The model under review builds one solid part; all positions refer to its coordinate system, in mm. Round coordinates to 2 decimals unless told otherwise and drop trailing zeros. Order: outer loops, then holes, each group sorted by start corner. A loop starts at its lowest first (then second) coordinate and runs counter-clockwise, first axis right, second up. Notation, with made-up numbers: M 45.5,81 L 91.5,81 A23 cw 91.5,105 Z; hole C -33.5,-18.5 d4. An arc over 180 degrees is marked long. Answer as a JSON object with one key per item and string values. Group by question number.
1. Add section A-A on x = 0. State the section outline as (y, z) points.
2. Add section D-D on z = 11.5. State the section outline as (x, y) points, and give its area (3 significant figures).
3. Add section B-B on y = 7. State the section outline as (x, z) points.
4. Clearance check with a flat-ended pin moving along its axis: P1, Ø4, axis at x = 0, z = -20, coming from the +Y side. State where the tip first meets the part, or that it passes through.
5. To check wall thickness, follow probe 1 along Z at (x, y) = (0, 7.8); probe 2 along Z at (x, y) = (0, 3.3); probe 3 along Y at (x, z) = (-5.75, -29.5). State the ranges of each line that lie inside material, in increasing order. Write a range as [from, to].
Autodesk Inventor part; units mm, degrees
ref_plane "to_block_XY" through (0, 9.5, 0) normal (0, 0, 1) x (1, 0, 0)
ref_plane "to_block_YZ" through (0, 9.5, 0) normal (1, 0, 0) x (0, 1, 0)
ref_plane "to_block_ZX" through (0, 9.5, 0) normal (0, 1, 0) x (0, 0, 1)
sketch "Sketch_12" plane through (0, 0, 0) normal (0, 0, 1) x (1, 0, 0)
  line L0 (-7.5, 9.2) -> (-7.5, 8.7239)
  line L1 (-7.5, 8.7239) -> (-6.94, 8.4006)
  arc A0 (-6.2177, 7.6) -> (-6.94, 8.4006) centre (-7.815, 6.885) ccw
  line L2 (-6.2177, 7.6) -> (-5, 7.6)
  line L3 (-5, 7.6) -> (-5, 6.4)
  line L4 (-5, 6.4) -> (-6.2177, 6.4)
  arc A1 (-6.94, 5.5994) -> (-6.2177, 6.4) centre (-7.815, 7.115) ccw
  line L5 (-6.94, 5.5994) -> (-7.5, 5.2762)
  line L6 (-7.5, 5.2762) -> (-7.5, 0.5)
  line L7 (-7.5, 0.5) -> (-7, 0)
  line L8 (-7, 0) -> (7, 0)
  line L9 (7, 0) -> (7.5, 0.5)
  line L10 (7.5, 0.5) -> (7.5, 5.2762)
  line L11 (7.5, 5.2762) -> (6.94, 5.5994)
  arc A2 (6.2177, 6.4) -> (6.94, 5.5994) centre (7.815, 7.115) ccw
  line L12 (6.2177, 6.4) -> (5, 6.4)
  line L13 (5, 6.4) -> (5, 7.6)
  line L14 (5, 7.6) -> (6.2177, 7.6)
  arc A3 (6.94, 8.4006) -> (6.2177, 7.6) centre (7.815, 6.885) ccw
  line L15 (6.94, 8.4006) -> (7.5, 8.7239)
  line L16 (7.5, 8.7239) -> (7.5, 9.2)
  line L17 (7.5, 9.2) -> (7.2, 9.5)
  line L18 (7.2, 9.5) -> (-7.2, 9.5)
  line L19 (-7.2, 9.5) -> (-7.5, 9.2)
extrude "Extrusion1" add sketch "Sketch_12" along normal mid plane 70
sketch "Sketch2" plane through (-7.2, 9.5, 35) normal (0, 1, 0) x (1, 0, 0)
  point P0 (7.2, 55)
hole "Hole1" at (0, 9.5, -20) direction (0, -1, 0) diameter 3.5 depth 9.5 counterbore diameter 6 counterbore depth 4.5
pattern_linear "Rectangular Pattern1" count 2 spacing 40 along (0, 0, 1) of "Hole1"
ref_plane "to_block_XY" through (0, 9.5, 0) normal (0, 0, 1) x (1, 0, 0)
ref_plane "to_block_YZ" through (0, 9.5, 0) normal (1, 0, 0) x (0, 1, 0)
ref_plane "to_block_ZX" through (0, 9.5, 0) normal (0, 1, 0) x (0, 0, 1)
properties part number "SSEBZ-MX16-70_r"
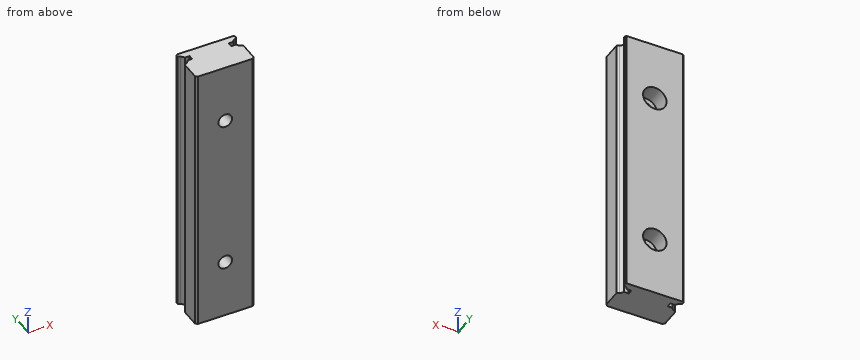
Recorded:
{
 "1": {"outline": "M 0,-35 L 9.5,-35 L 9.5,-23 L 5,-23 L 5,-21.75 L 0,-21.75 Z; M 0,-18.25 L 5,-18.25 L 5,-17 L 9.5,-17 L 9.5,17 L 5,17 L 5,18.25 L 0,18.25 Z; M 0,21.75 L 5,21.75 L 5,23 L 9.5,23 L 9.5,35 L 0,35 Z"},
 "2": {"outline": "M -7.5,0.5 L -7,0 L 7,0 L 7.5,0.5 L 7.5,5.28 L 6.94,5.6 A1.75 cw 6.22,6.4 L 5,6.4 L 5,7.6 L 6.22,7.6 A1.75 cw 6.94,8.4 L 7.5,8.72 L 7.5,9.2 L 7.2,9.5 L -7.2,9.5 L -7.5,9.2 L -7.5,8.72 L -6.94,8.4 A1.75 cw -6.22,7.6 L -5,7.6 L -5,6.4 L -6.22,6.4 A1.75 cw -6.94,5.6 L -7.5,5.28 Z", "area": "133 mm²"},
 "3": {"outline": "M -5,-35 L 5,-35 L 5,35 L -5,35 Z; hole C 0,-20 d6; hole C 0,20 d6"},
 "4": {"P1": "stops at y = 5"},
 "5": {"probe 1": "z = [-35, -23], [-17, 17], [23, 35]", "probe 2": "z = [-35, -21.75], [-18.25, 18.25], [21.75, 35]", "probe 3": "y = [0, 6.4], [7.6, 9.5]"}
}
